For this review, take the finished solid that the model builds, in its own axes (mm). A direction names the side the tool comes from. Coordinates: 2 decimals unless noted, no trailing zeros. Order: outer loops, then holes, each group sorted by start corner. A loop starts at its lowest first (then second) coordinate and runs counter-clockwise, first axis right, second up. Notation, with made-up numbers: (30, 1.25) - (39, 1.25) arc R25 ccw to (39, 36.25) - close; hole circle Ø11 at (42.25, 86). An arc over 180 degrees is marked (long way). One line per item, written item: value. Start each with the question number.
(1) Consider section B-B on x = -28. Write out the cut boundary in (y, z).
(2) Clearance check with a flat-ended pin moving along its axis: pin 1 (3 mm diameter, centred on x = -13, y = 54, fed in from +Z). State where the tip first meets the part, or that it passes through.
(3) To check wall thickness, follow line 1 along Y through (x, z) = (-4.5, 13.75); line 2 along Y through (x, z) = (-16, 11.5); line 3 along X through (y, z) = (81.5, 15). State the ranges of each line that lie inside material, in increasing order.
(4) Mouldability with a two-part tool opening along X and no side actions: class faces 3 (the flat face through (-56, 59, 15)), 4 (the flat face through (-3, 35, 16)), 5 (the flat face through (-28, 0, 15)) as released by +X, released by -X, zero draft, split by the parting line, or undercut.
(5) For faces 1 (the flat face through (-28, 61, 0)), 2 (the flat face through (-12, 116, 29)), list the 3-axis set-ups (+Z, -Z, +X, -X, +Y, -Y) from which the entire face can be reached by the end or side of a thin tool; tool diameter is ignored.
(6) Consider section D-D on x = -34. Write out the cut boundary in (y, z), then the cut area to 3 significant figures.
(7) Consider section C-C on y = 91. Write out the cut boundary in (x, z), then the cut area to 3 significant figures.
(8) Consider section A-A on z = 11. Write out the cut boundary in (x, y).
```python
from build123d import *

# Parameters (mm, degrees)
SKETCH1_W           = 56
SKETCH1_H           = 120
BOSS_EXTRUDE1_DEPTH = 30
SHELL1_T            = -3
SKETCH2_W           = 50
SKETCH2_H           = 3
BOSS_EXTRUDE2_DEPTH = 26
CUT_EXTRUDE5_DEPTH  = 3
SKETCH6_W           = 30
SKETCH6_H           = 2
BOSS_EXTRUDE3_DEPTH = 3
SKETCH7_W           = 30
SKETCH7_H           = 2
BOSS_EXTRUDE4_DEPTH = 3


with BuildPart() as part:
    # Sketch1 → Boss-Extrude1 (new body)
    with BuildSketch(Plane.XY):
        with Locations((-28, 60)):
            Rectangle(SKETCH1_W, SKETCH1_H)
    extrude(amount=BOSS_EXTRUDE1_DEPTH)

    # Shell1
    shell1_openings = [part.faces().sort_by_distance(p)[0] for p in [
        (-28, 60, 30),
    ]]
    offset(amount=SHELL1_T, openings=shell1_openings, kind=Kind.INTERSECTION)

    # Sketch2 → Boss-Extrude2 (add)
    with BuildSketch(Plane.XY.offset(3)):
        with Locations((-28, 115.5)):
            Rectangle(SKETCH2_W, SKETCH2_H)
    extrude(amount=BOSS_EXTRUDE2_DEPTH)

    # Sketch3 → Cut-Extrude5 (cut)
    with BuildSketch(Plane.XZ.offset(-114)):
        with BuildLine():
            Line((-36, 29), (-20, 29))
            ThreePointArc((-20, 29), (-28, 21), (-36, 29))
        make_face()
    extrude(amount=-CUT_EXTRUDE5_DEPTH, mode=Mode.SUBTRACT)

    # Sketch6 → Boss-Extrude3 (add)
    with BuildSketch(Plane(origin=(-53, 0, 0), x_dir=(0, 0, -1), z_dir=(1, 0, 0))):
        with Locations((-15, 73)):
            Rectangle(SKETCH6_W, SKETCH6_H)
    boss_extrude3 = extrude(amount=BOSS_EXTRUDE3_DEPTH)

    # Sketch7 → Boss-Extrude4 (add)
    with BuildSketch(Plane(origin=(-53, 0, 0), x_dir=(0, 0, -1), z_dir=(1, 0, 0))):
        with Locations((-15, 69)):
            Rectangle(SKETCH7_W, SKETCH7_H)
    boss_extrude4 = extrude(amount=BOSS_EXTRUDE4_DEPTH)

    # Mirror1: Boss-Extrude3, Boss-Extrude4 across plane
    add(boss_extrude3.mirror(Plane(origin=(-28, 0, 0), x_dir=(0, 0, 1), z_dir=(1, 0, 0))))
    add(boss_extrude4.mirror(Plane(origin=(-28, 0, 0), x_dir=(0, 0, 1), z_dir=(1, 0, 0))))


solid = part.part
```
Geometry check:
1. outline: (0, 0) - (120, 0) - (120, 30) - (117, 30) - (117, 21) - (114, 21) - (114, 3) - (3, 3) - (3, 30) - (0, 30) - close
2. pin 1: stops at z = 3
3. line 1: y = 0 to 3, 68 to 70, 72 to 74, 114 to 120
3. line 2: y = 0 to 3, 114 to 120
3. line 3: x = -56 to -53, -3 to 0
4. face 3: released by -X
4. face 4: undercut
4. face 5: zero draft
5. face 1: -Z, +X, -X, +Y, -Y
5. face 2: +Z
6. outline: (0, 0) - (120, 0) - (120, 30) - (117, 30) - (117, 23.71) - (114, 23.71) - (114, 3) - (3, 3) - (3, 30) - (0, 30) - close
6. area: 584 mm^2
7. outline: (-56, 0) - (0, 0) - (0, 30) - (-3, 30) - (-3, 3) - (-53, 3) - (-53, 30) - (-56, 30) - close
7. area: 330 mm^2
8. outline: (-56, 0) - (0, 0) - (0, 120) - (-56, 120) - close; hole (-53, 3) - (-3, 3) - (-3, 68) - (-6, 68) - (-6, 70) - (-3, 70) - (-3, 72) - (-6, 72) - (-6, 74) - (-3, 74) - (-3, 114) - (-53, 114) - (-53, 74) - (-50, 74) - (-50, 72) - (-53, 72) - (-53, 70) - (-50, 70) - (-50, 68) - (-53, 68) - close
